from build123d import *

# Parameters (mm, degrees)
F1_DEPTH = 12.7
F3_D     = 4.318
F3_DEPTH = 25.4
F3_TIP   = 1.2972580765


with BuildPart() as f1:
    # F0 (on Front) → F1 (new body)
    with BuildSketch(Plane.XZ):
        with BuildLine():
            ThreePointArc((0, 57.15), (24.1526336585, 51.7954900291), (43.7794399242, 36.7353118936))
            Line((43.7794399242, 36.7353118936), (45.7251928098, 38.3679924222))
            ThreePointArc((45.7251928098, 38.3679924222), (42.1021507188, 42.3119959923), (38.1401829521, 45.9153846154))
            ThreePointArc((38.1401829521, 45.9153846154), (36.2252205848, 52.95698775), (42.1976492236, 57.15))
            Line((42.1976492236, 57.15), (76.2, 57.15))
            Line((76.2, 57.15), (76.2, 59.69))
            Line((76.2, 59.69), (0, 59.69))
            ThreePointArc((0, 59.69), (-25.2260840433, 54.0975118082), (-45.7251928098, 38.3679924222))
            Line((-45.7251928098, 38.3679924222), (-43.7794399242, 36.7353118936))
            ThreePointArc((-43.7794399242, 36.7353118936), (-24.1526336585, 51.7954900291), (0, 57.15))
        make_face()
        with BuildLine():
            Line((17.2271181571, 57.15), (35.975945277, 57.15))
            ThreePointArc((35.975945277, 57.15), (33.7657449416, 53.6169292109), (33.4084844583, 49.4648285775))
            ThreePointArc((33.4084844583, 49.4648285775), (25.6077435165, 53.9178965836), (17.2271181571, 57.15))
        make_face(mode=Mode.SUBTRACT)
    extrude(amount=F1_DEPTH)

    # F3
    with Locations(Plane(origin=(0, 0, 57.15), x_dir=(1, 0, 0), z_dir=(0, 0, -1))):
        with Locations((69.85, 6.35), (50.8, 6.35)):
            Hole(F3_D / 2, depth=F3_DEPTH)
            with Locations((0, 0, -(F3_DEPTH + F3_TIP / 2))):  # 118° drill point
                Cone(0, F3_D / 2, F3_TIP, mode=Mode.SUBTRACT)


solid = f1.part
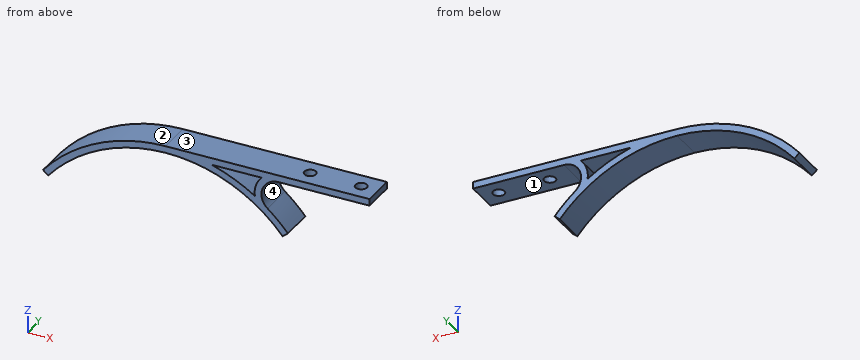
Geometry check sheet. Reference: the model listing, model coordinates, mm. Face numbers are marked on the shaded views. A direction names the side the tool comes from. Coordinates: 2 decimals unless noted, no trailing zeros. Order: outer loops, then holes, each group sorted by start corner. A loop starts at its lowest first (then second) coordinate and runs counter-clockwise, first axis right, second up. Notation, with made-up numbers: (-24.5, 75.25) -> (22.5, 75.25) arc R10 ccw to (22.5, 92.25) -> close; hole circle Ø8 at (87.5, 26.5). An arc over 180 degrees is marked (long way). Use a Markdown table: item, result. Add a question column.
1. Material ranges on L1, parallel to X at y = -9.5, z = 49.75; L2, parallel to Y at x = 50.8, z = 58.9; L3, parallel to Z at x = 18, y = -1.75, recorded low to high.
2. Set-up check for the marked faces 1 and 2: record each of +Z, -Z, +X, -X, +Y, -Y from which the full face is reachable in a straight line by a thin tool's end or side.
3. Go/stop test with flat-tipped pins: pin 1 Ø5 at (y, z) = (-7.5, 43.5) entering from +X; pin 2 Ø4 at (y, z) = (-2.5, 48.5) entering from +X; pin 3 Ø4 at (x, y) = (-8, -4) entering from +Z; pin 4 Ø4 at (x, y) = (69.85, -6.35) entering from -Z. Record where each tip stops, or that it passes through.
4. Cross-section at C-C (x = 50.8). Enter the section's corners in (y, z).
5. Cross-section at D-D (x = -38). Enter the section's corners in (y, z).
6. Cross-section at A-A (y = -6.35). Enter the section's corners in (x, z), and give its area (3 significant figures).
7. Mould release check, pull along Z, two halves, no side actions. Record for the marked faces 3 and 4: pulls with the +Z half, pulls with the -Z half, needs draft (parallel to the pull), parting line crosses it, or undercut.
8. Cross-section at B-B (z = 41). Enter the section's corners in (x, y).
Filled sheet:
| question | item | result |
|---|---|---|
| 1 | L1 | -32.98 to -28.13, 28.13 to 32.98, 33.37 to 35.94 |
| 1 | L2 | -12.7 to -8.51, -4.19 to 0 |
| 1 | L3 | 54.24 to 56.91, 57.15 to 59.69 |
| 2 | face 1 | +X, +Y, -Y |
| 2 | face 2 | +Z, -X, +Y, -Y |
| 3 | pin 1 | x = 43.38 |
| 3 | pin 2 | x = 37.53 |
| 3 | pin 3 | z = 59.39 |
| 3 | pin 4 | through |
| 4 | outline | (-12.7, 57.15) -> (-8.51, 57.15) -> (-8.51, 59.69) -> (-12.7, 59.69) -> close; (-4.19, 57.15) -> (0, 57.15) -> (0, 59.69) -> (-4.19, 59.69) -> close |
| 5 | outline | (-12.7, 42.69) -> (0, 42.69) -> (0, 46.03) -> (-12.7, 46.03) -> close |
| 6 | outline | (-45.73, 38.37) -> (-43.78, 36.74) arc R57.15 cw to (43.78, 36.74) -> (45.73, 38.37) arc R59.69 ccw to (38.14, 45.92) arc R6.35 cw to (42.2, 57.15) -> (48.64, 57.15) -> (48.64, 59.69) -> (0, 59.69) arc R59.69 ccw to start; (52.96, 57.15) -> (67.69, 57.15) -> (67.69, 59.69) -> (52.96, 59.69) -> close; (72.01, 57.15) -> (76.2, 57.15) -> (76.2, 59.69) -> (72.01, 59.69) -> close; hole (17.23, 57.15) arc R59.69 cw to (33.41, 49.46) arc R8.89 cw to (35.98, 57.15) -> close |
| 6 | area | 428 mm2 |
| 7 | face 3 | pulls with the +Z half |
| 7 | face 4 | undercut |
| 8 | outline | (-43.38, -12.7) -> (-39.81, -12.7) -> (-39.81, 0) -> (-43.38, 0) -> close; (39.81, -12.7) -> (43.38, -12.7) -> (43.38, 0) -> (39.81, 0) -> close |
